For this review, take the finished solid that the model builds, in its own axes (mm). Give positions to 0.01 mm unless a question says otherwise; leave off trailing zeros. Order: outer loops, then holes, each group sorted by start corner. A loop starts at its lowest first (then second) coordinate and runs counter-clockwise, first axis right, second up. Notation, with made-up numbers: (81, -4.5) -> (102, -4.5) arc R16 ccw to (102, -0.5) -> close; hole circle Ø2 at (-34, 55). An arc over 180 degrees is marked (long way). Use CSV: the item, a comma, the result in double quotes. Start each with the question number.
```python
from build123d import *

# Parameters (mm, degrees)
SKETCH1_R           = 6
SKETCH1_R_2         = 2
BOSS_EXTRUDE1_DEPTH = 1
CUT_EXTRUDE1_DEPTH  = 9.544003745


with BuildPart() as part:
    # Sketch1 → Boss-Extrude1 (new body)
    with BuildSketch(Plane(origin=(0, 0, 0), x_dir=(1, 0, 0), z_dir=(0, 1, 0))):
        with Locations(Location((0, 0, 0), (0, 0, 270))):
            Circle(SKETCH1_R)
        with Locations(Location((0, 0, 0), (0, 0, 270))):
            Circle(SKETCH1_R_2, mode=Mode.SUBTRACT)
    extrude(amount=BOSS_EXTRUDE1_DEPTH)

    # Sketch2 → Cut-Extrude1 (cut, through all)
    with BuildSketch(Plane(origin=(0, 1, 0), x_dir=(1, 0, 0), z_dir=(0, 1, 0))):
        with BuildLine():
            Line((-5, -3.31662479), (-5, 3.31662479))
            ThreePointArc((-5, 3.31662479), (-6, 0), (-5, -3.31662479))
        make_face()
        with BuildLine():
            Line((5, 3.31662479), (5, -3.31662479))
            ThreePointArc((5, -3.31662479), (6, 0), (5, 3.31662479))
        make_face()
    extrude(amount=-CUT_EXTRUDE1_DEPTH, mode=Mode.SUBTRACT)


solid = part.part
```
1. Consider section A-A (x = 0). State the section outline as (y, z) points, plus the area to 3 significant figures.
2. Draft analysis for pull direction X (two halves, no side actions). For faces 1 (the face through (5, 0.5, 0)), 2 (the face through (-1.952, 0.493, -0.434)), 3 (the face through (0.1, 0.5, -6)), state which applies: +X half, -X half, draft (parallel to the pull), parting line (faces both ways), or undercut.
3. Clearance check with a flat-ended pin moving along its axis: P1, Ø2.5, axis at x = 0, z = 0, coming from the -Y side. State where the tip first meets the part, or that it passes through.
4. Consider section D-D (x = -2.5). State the section outline as (y, z) points, plus the area to 3 significant figures.
5. Consider section C-C (y = 0.4). State the section outline as (x, z) points.
6. Consider section B-B (z = 0). State the section outline as (x, y) points.
7. To check wall thickness, follow L1, parallel to X at y = 0.3, z = 0; L2, parallel to Z at x = 0.25, y = 0.25; L3, parallel to X at y = 0.25, z = 1.25. State the ranges of each line that lie inside material, in increasing order. Write a range as [from, to].
Answer list:
1,outline,"(0, -6) -> (1, -6) -> (1, -2) -> (0, -2) -> close; (0, 2) -> (1, 2) -> (1, 6) -> (0, 6) -> close"
1,area,"8.00 mm2"
2,face 1,"+X half"
2,face 2,"undercut"
2,face 3,"parting line"
3,P1,"through"
4,outline,"(0, -5.45) -> (1, -5.45) -> (1, 5.45) -> (0, 5.45) -> close"
4,area,"10.9 mm2"
5,outline,"(-5, -3.32) arc R6 ccw to (5, -3.32) -> (5, 3.32) arc R6 ccw to (-5, 3.32) -> close; hole circle Ø4 at (0, 0)"
6,outline,"(-5, 0) -> (-2, 0) -> (-2, 1) -> (-5, 1) -> close; (2, 0) -> (5, 0) -> (5, 1) -> (2, 1) -> close"
7,L1,"[-5, -2], [2, 5]"
7,L2,"[-5.99, -1.98], [1.98, 5.99]"
7,L3,"[-5, -1.56], [1.56, 5]"
